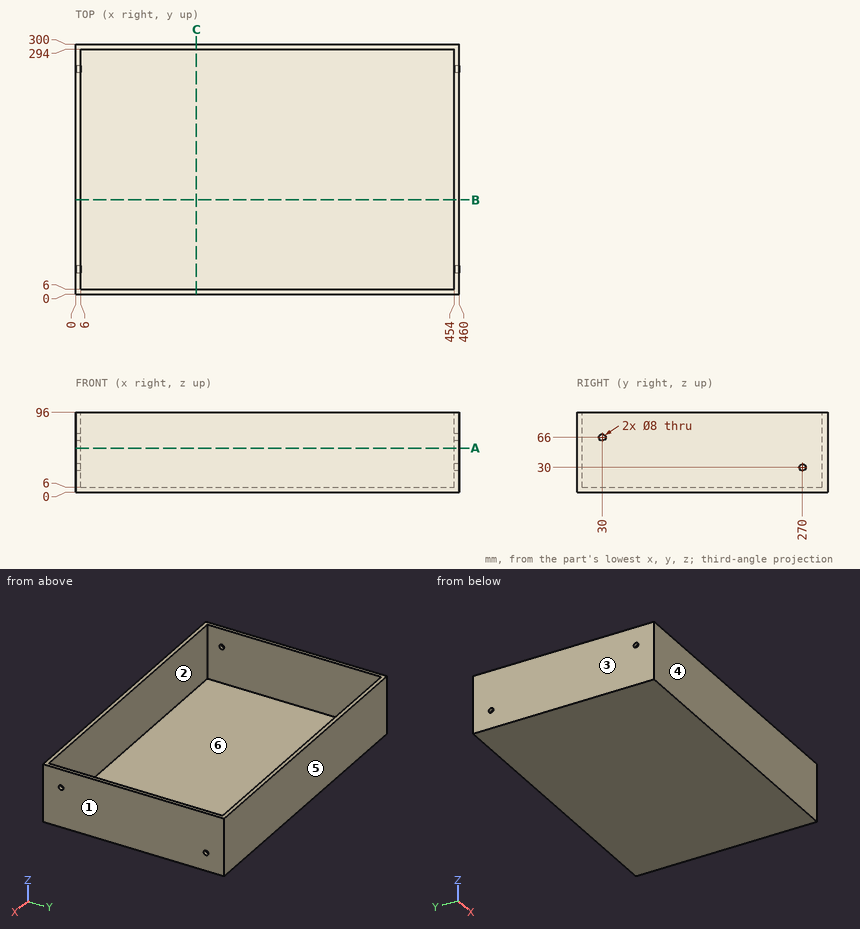
Answer from the drawing. Dimensions are ordinates in mm from the lowest x, y and z of the part. A direction names the side the tool comes from. Round coordinates to 2 decimals unless told otherwise and drop trailing zeros. Loops run counter-clockwise (first coordinate to the right, second up) from the corner with the lowest first, then second, coordinate; pieces in that order, holes last.
(1) The part is cut by section C-C, the plane x = 145. Give the vertices of the cut face in (y, z).
Computed values:
outline: (0, 0) - (300, 0) - (300, 96) - (294, 96) - (294, 6) - (6, 6) - (6, 96) - (0, 96) - close
(2) This flat-tipped pin is pushed along its axis until it touches: P1, Ø2, axis at x = 181, y = 177, coming from the +Z side. Where does it stop, or does it pass through?
Computed values:
P1: stops at z = 6
(3) The part is cut by section B-B, the plane y = 113. Give the vertices of the cut face in (x, z), and give its area (3 significant figures).
Computed values:
outline: (0, 0) - (460, 0) - (460, 96) - (454, 96) - (454, 6) - (6, 6) - (6, 96) - (0, 96) - close
area: 3,840 mm2
(4) The mould has two halves that part along X. Classify the marked faces 1, 2, 3 and 4: pulls with the +X half, pulls with the -X half, needs draft (parallel to the pull), parting line crosses it, or undercut.
Computed values:
face 1: pulls with the +X half
face 2: undercut
face 3: pulls with the -X half
face 4: needs draft
(5) The part is cut by section A-A, the plane z = 53. Give the vertices of the cut face in (x, y), and give its area (3 significant figures).
Computed values:
outline: (0, 0) - (460, 0) - (460, 300) - (0, 300) - close; hole (6, 6) - (454, 6) - (454, 294) - (6, 294) - close
area: 8,980 mm2
(6) Find the intervals of material crossed by L1, parallel to Y at x = 367, z = 51.5; L2, parallel to X at y = 111, z = 36; L3, parallel to Z at x = 457, y = 30, in increasing order.
Computed values:
L1: y = 0 to 6, 294 to 300
L2: x = 0 to 6, 454 to 460
L3: z = 0 to 62, 70 to 96
(7) For the marked faces 5 and 6, determine the directions among +Z, -Z, +X, -X, +Y, -Y from which every point of the face is accessible in a straight line to the end or side of a thin tool.
Computed values:
face 5: +Z, -Z, +X, -X, +Y
face 6: +Z
